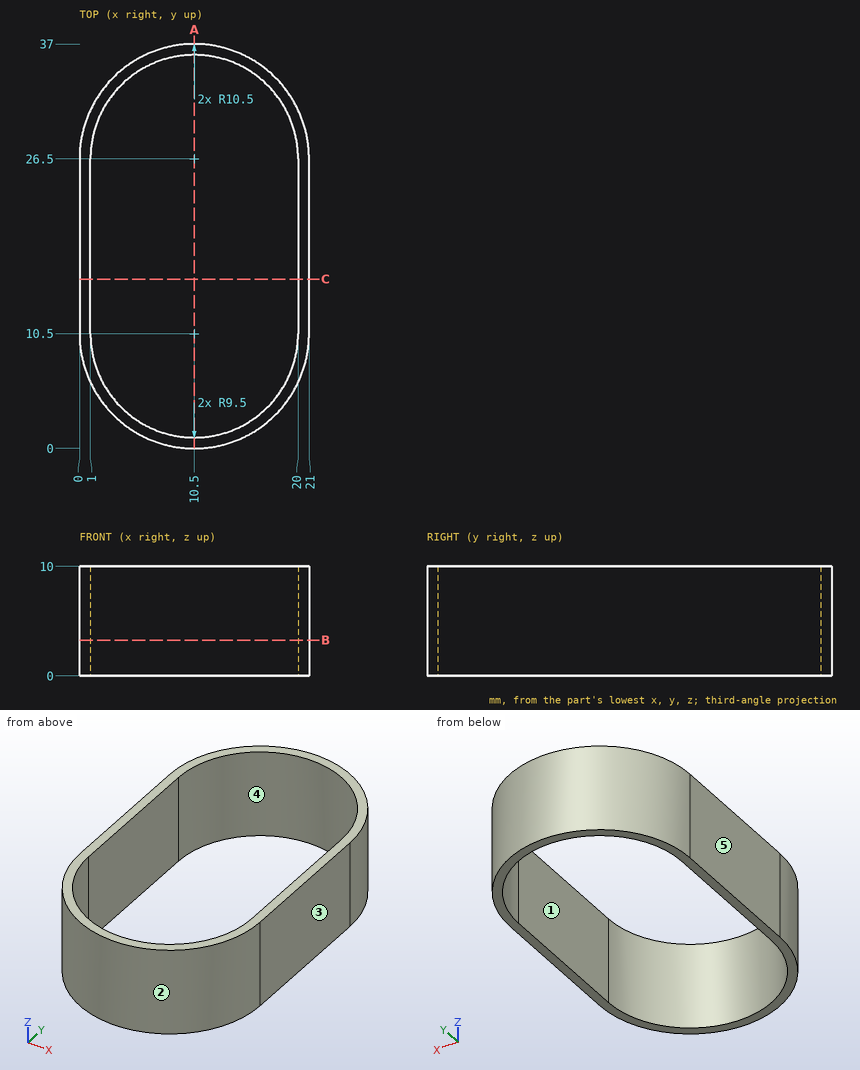
Geometry: see drawing. Coordinates: mm, zero at the bounding-box minimum. A direction names the side the tool comes from. Round coordinates to 2 decimals unless told otherwise and drop trailing zeros. Loops run counter-clockwise (first coordinate to the right, second up) from the corner with the lowest first, then second, coordinate; pieces in that order, holes last. Notation, with made-up numbers: (33, -29.5) -> (66, -29.5) arc R21 cw to (66, -6.5) -> close; hole circle Ø10 at (-12.5, 33). An arc over 180 degrees is marked (long way). Write each question's results on one line, items separated by ' | '.
Item 1: Pull-direction query (X, two-part tool) for the marked faces 3, 4 and 5; classes: pulls with the +X half, pulls with the -X half, needs draft (parallel to the pull), parting line crosses it, or undercut.
Answers below:
face 3: pulls with the +X half | face 4: undercut | face 5: pulls with the -X half
Item 2: Pin query (flat end, axial travel): pin 1 Ø6 at (y, z) = (30, 5) entering from +X; pin 2 Ø2 at (x, z) = (16.5, 2.5) entering from +Y; pin 3 Ø3 at (x, z) = (17, 3) entering from -Y; pin 4 Ø12 at (x, y) = (3.5, 15.5) entering from +Z. Return the tip coordinate at first contact, or that it passes through.
Answers below:
pin 1: stops at x = 20.99 | pin 2: stops at y = 35.73 | pin 3: stops at y = 1.27 | pin 4: stops at z = 10
Item 3: Cut plane C-C on y = 15.5. Return the cut outline in (x, z).
Answers below:
outline: (0, 0) -> (1, 0) -> (1, 10) -> (0, 10) -> close; (20, 0) -> (21, 0) -> (21, 10) -> (20, 10) -> close
Item 4: Set-up query: the marked faces 1 and 2. Return all of +Z, -Z, +X, -X, +Y, -Y with unobstructed straight access to the full face (end or side cutting, diameter ignored); none if empty.
Answers below:
face 1: +Z, -Z | face 2: +Z, -Z, -Y
Item 5: Line query: probe 1 along Y at (x, z) = (10.5, 1.5); probe 2 along X at (y, z) = (22, 5.75); probe 3 along Y at (x, z) = (4.5, 5.5). Output: solid intervals per line, ascending. Write a range as [from, to].
Answers below:
probe 1: y = [0, 1], [36, 37] | probe 2: x = [0, 1], [20, 21] | probe 3: y = [1.88, 3.13], [33.87, 35.12]
Item 6: Cut plane A-A on x = 10.5. Return the cut outline in (y, z).
Answers below:
outline: (0, 0) -> (1, 0) -> (1, 10) -> (0, 10) -> close; (36, 0) -> (37, 0) -> (37, 10) -> (36, 10) -> close
Item 7: Cut plane B-B on z = 3.25. Return the cut outline in (x, y), and give its area (3 significant figures).
Answers below:
outline: (0, 10.5) arc R10.5 ccw to (21, 10.5) -> (21, 26.5) arc R10.5 ccw to (0, 26.5) -> close; hole (1, 10.5) arc R9.5 ccw to (20, 10.5) -> (20, 26.5) arc R9.5 ccw to (1, 26.5) -> close | area: 94.8 mm²
